Verification items for the finished model (mm, model axes). Coordinates: 2 decimals unless noted, no trailing zeros. Order: outer loops, then holes, each group sorted by start corner. A loop starts at its lowest first (then second) coordinate and runs counter-clockwise, first axis right, second up. Notation, with made-up numbers: M -32.75,69.25 L 5.25,69.25 A30 cw 5.25,108.25 Z; hole C 82,-21.5 d7. An arc over 180 degrees is marked long. Return JSON: item names as keys, results as strings. Group by question number.
Q1. Go/stop test with flat-tipped pins: pin 1 Ø1 at (x, y) = (2, 9.5) entering from +Z; pin 2 Ø1.5 at (y, z) = (3.5, -1) entering from +X; pin 3 Ø1.5 at (x, y) = (-2, 17) entering from +Z. Record where each tip stops, or that it passes through.
Q2. Thickness scan on probe 1 along Y at (x, z) = (2.1, -1.6); probe 2 along Z at (x, y) = (2.55, 23); probe 3 along Z at (x, y) = (-1.95, 6). Record the ranges inside material, lowest first.
Q3. Section check A-A, the plane y = 22.75. Enter the section's corners in (x, z).
from build123d import *

# Parameters (mm, degrees)
BOSS_EXTRUDE1_DEPTH   = 25
CHAMFER1_SIZE2        = 0.500023177
CHAMFER1_SIZE         = 0.500027299
CHAMFER1_EDGE_2_SIZE2 = 0.500023177
CHAMFER1_EDGE_2_SIZE  = 0.500027299


with BuildPart() as part:
    # Sketch1 → Boss-Extrude1 (new body)
    with BuildSketch(Plane(origin=(0, 25, 0), x_dir=(1, 0, 0), z_dir=(0, 1, 0))):
        with BuildLine():
            Line((1.077032961, 2.8), (-1.077032961, 2.8))
            ThreePointArc((-1.077032961, 2.8), (0, -3), (1.077032961, 2.8))
        make_face()
    extrude(amount=-BOSS_EXTRUDE1_DEPTH)

    # Chamfer1
    chamfer1_edges = [part.edges().sort_by_distance(p)[0] for p in [
        (0, 25, -2.8),
    ]]
    chamfer(chamfer1_edges, length=CHAMFER1_SIZE, length2=CHAMFER1_SIZE2)

    # Chamfer1 edge 2
    chamfer1_edge_2_edges = [part.edges().sort_by_distance(p)[0] for p in [
        (0, 25, 3),
    ]]
    chamfer(chamfer1_edge_2_edges, length=CHAMFER1_EDGE_2_SIZE, length2=CHAMFER1_EDGE_2_SIZE2)


solid = part.part
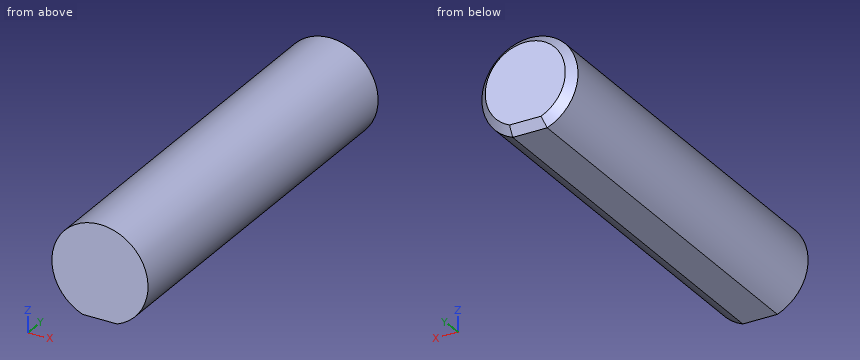
Numbers:
{
 "1": {"pin 1": "stops at z = 2.6", "pin 2": "stops at x = 2.99", "pin 3": "stops at z = 2.73"},
 "2": {"probe 1": "y = 0 to 24.86", "probe 2": "z = -1.58 to 1.58", "probe 3": "z = -2.28 to 2.28"},
 "3": {"outline": "M -1.08,-2.8 L 1.08,-2.8 A3 ccw long Z"}
}
